Build history of the part. All positions in model axes, mm. Face numbers are marked on the shaded views. Round coordinates to 2 decimals unless told otherwise and drop trailing zeros. Write each loop counter-clockwise with the first axis right and the second up, starting at its lowest first coordinate (ties: lowest second). Pieces come first, ordered by that corner, then holes. Notation, with made-up numbers: (67, -17.5) -> (122, -17.5) arc R10 ccw to (122, -8.5) -> close; hole circle Ø2 at (53, 63.25). An arc over 180 degrees is marked (long way). One line per question, with ' | ' between items.
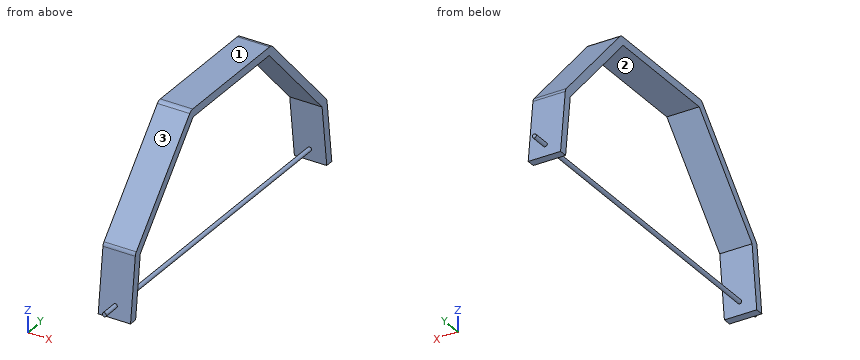
from build123d import *

# Parameters (mm, degrees)
F1_DEPTH = 12.7
F2_R     = 5.08
F3_R     = 1.5875
F4_DEPTH = 254
F5_R     = 1.5875
F6_DEPTH = 139.7


with BuildPart() as f1:
    # F0 (on Right) → F1 (new body, symmetric)
    with BuildSketch(Plane.YZ):
        Polygon((-120.803595, 50.8), (-127, 0), (-120.60294, 0), (-114.747306, 48.006249), (-48.010771, 120.650004), (0, 120.650004), (48.010771, 120.650004), (114.747306, 48.006249), (120.60294, 0), (127, 0), (120.803595, 50.8), (50.8, 127), (0, 127), (-50.8, 127), align=None)
    extrude(amount=F1_DEPTH, both=True)

    # F2
    f2_edges = [f1.edges().sort_by_distance(p)[0] for p in [
        (0, -120.803595, 50.8),
        (0, 120.803595, 50.8),
        (0, -50.8, 127),
        (0, 50.8, 127),
    ]]
    fillet(f2_edges, radius=F2_R)

    # F3 (on Front) → F4 (cut, symmetric)
    with BuildSketch(Plane.XZ):
        with Locations((0, 9.525)):
            Circle(F3_R)
    extrude(amount=F4_DEPTH, both=True, mode=Mode.SUBTRACT)

    # F5 (on Front) → F6 (join, symmetric)
    with BuildSketch(Plane.XZ):
        with Locations((0, 9.525)):
            Circle(F5_R)
    extrude(amount=F6_DEPTH, both=True)


solid = f1.part
(1) Mould opens along Y. For the marked faces 1, 2 and 3 say: pulls with the +Y half, pulls with the -Y half, needs draft (parallel to the pull), parting line crosses it, or undercut.
Calculated:
face 1: needs draft | face 2: undercut | face 3: pulls with the -Y half
(2) Slice it at C-C (y = 70). Write the cut outline in (x, z) (1 decimal), then the cut area to 3 significant figures.
Calculated:
outline: (-12.7, 96.7) -> (12.7, 96.7) -> (12.7, 106.1) -> (-12.7, 106.1) -> close; circle Ø3.2 at (0, 9.5) | area: 246 mm2
(3) Wall check: line 1 (Y direction, x = 11.25, z = 109.5); line 2 (Y direction, x = 11.25, z = 85.5); line 3 (Z direction, x = 4.5, y = -2.5). Give the ranges that are in metal, low to high. Write a range as from..to.
Calculated:
line 1: -66.88..-58.25, 58.25..66.88 | line 2: -88.93..-80.3, 80.3..88.93 | line 3: 120.65..127
(4) Slice it at B-B (x = -8). Write the cut outline in (y, z) (3 decimals).
Calculated:
outline: (-127, 0) -> (-120.603, 0) -> (-114.747, 48.006) -> (-48.011, 120.65) -> (48.011, 120.65) -> (114.747, 48.006) -> (120.603, 0) -> (127, 0) -> (121.001, 49.18) arc R5.08 ccw to (119.7, 52.002) -> (52.31, 125.357) arc R5.08 ccw to (48.569, 127) -> (-48.569, 127) arc R5.08 ccw to (-52.31, 125.357) -> (-119.7, 52.002) arc R5.08 ccw to (-121.001, 49.18) -> close
(5) Slice it at D-D (z = 99.5). Write the cut outline in (x, y), then the cut area to 3 significant figures.
Calculated:
outline: (-12.7, -76.06) -> (12.7, -76.06) -> (12.7, -67.44) -> (-12.7, -67.44) -> close; (-12.7, 67.44) -> (12.7, 67.44) -> (12.7, 76.06) -> (-12.7, 76.06) -> close | area: 438 mm2
(6) Drop flat-ended pins along their axis: pin 1 (3 mm diameter, centred on x = -5, z = 73.5, fed in from +Y); pin 2 (3 mm diameter, centred on x = 6.5, y = 52.5, fed in from +Z); pin 3 (5 mm diameter, centred on x = -1, y = 55.5, fed in from +Z); pin 4 (10 mm diameter, centred on y = -73.5, z = 86.5, fed in from +X). Give the stop position or say it passes through.
Calculated:
pin 1: y = 101.33 | pin 2: z = 126.38 | pin 3: z = 124.61 | pin 4: x = 12.7
(7) Slice it at A-A (z = 31.5). Write the cut outline in (x, y), then the cut area to 3 significant figures.
Calculated:
outline: (-12.7, -123.16) -> (12.7, -123.16) -> (12.7, -116.76) -> (-12.7, -116.76) -> close; (-12.7, 116.76) -> (12.7, 116.76) -> (12.7, 123.16) -> (-12.7, 123.16) -> close | area: 325 mm2
